The model under review builds one solid part; all positions refer to its coordinate system, in mm. Give positions to 0.01 mm unless a question says otherwise; leave off trailing zeros. Loops run counter-clockwise (first coordinate to the right, second up) from the corner with the lowest first, then second, coordinate; pieces in that order, holes last. Notation, with made-up numbers: (86.25, 21) -> (117.25, 21) arc R27 cw to (117.25, 60) -> close; hole circle Ø8 at (10, 67). An arc over 180 degrees is marked (long way). Write each question's results on one line, items separated by ' | '. Start each with the question number.
Q1. We need section B-B (x = 62). Write out the cut boundary in (y, z), plus the area to 3 significant figures.
Q2. Insertion check: pin 1 Ø1.8 at (y, z) = (-3.5, 5.5) entering from +X; pin 2 Ø3 at (x, y) = (133.5, -2) entering from -Z; pin 3 Ø2.5 at (y, z) = (-2.5, 222) entering from +X; pin 4 Ø6 at (x, z) = (76.5, 101.5) entering from +Y. Each pin has a flat end and moves straight along its axis. Give the tip position at first contact, or say it passes through.
Q3. Wall thickness on L1, parallel to X at y = -0.35, z = 2; L2, parallel to Z at x = 5, y = -3.1; L3, parallel to Z at x = 73, y = -4.35: over which ranges is each line inside the solid? List them lowest first. Write a range as [from, to].
Q4. We need section A-A (z = 106.5). Write out the cut boundary in (x, y), plus the area to 3 significant figures.
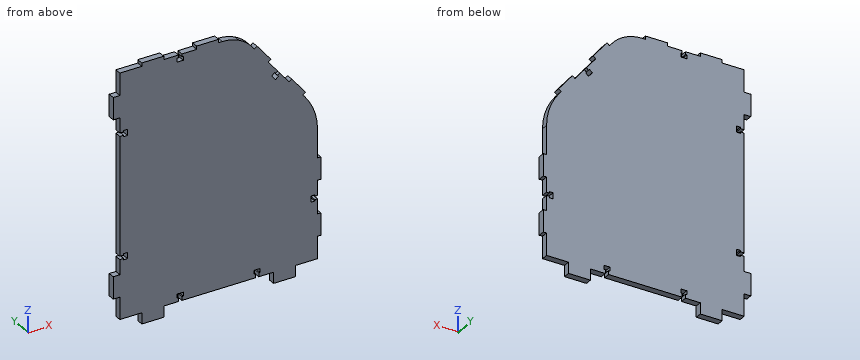
from build123d import *

# Parameters (mm, degrees)
F1_DEPTH = 6


# Not quite as in the source:
# - a feature names something its author has since deleted; it is built from what else it names


with BuildPart() as f1:
    # F0 (on Front) → F1 (new body)
    with BuildSketch(Plane.XZ):
        with BuildLine():
            Line((20, 220), (0, 220))
            Line((0, 220), (0, 200))
            Line((0, 200), (-6, 200))
            Line((-6, 200), (-6, 180))
            Line((-6, 180), (0, 180))
            Line((0, 180), (0, 166.5))
            Line((0, 166.5), (3.5, 166.5))
            Line((3.5, 166.5), (3.5, 167.75))
            Line((3.5, 167.75), (7, 167.75))
            Line((7, 167.75), (7, 162.25))
            Line((7, 162.25), (3.5, 162.25))
            Line((3.5, 162.25), (3.5, 163.5))
            Line((3.5, 163.5), (0, 163.5))
            Line((0, 163.5), (0, 110))
            Line((0, 110), (0, 56.5))
            Line((0, 56.5), (3.5, 56.5))
            Line((3.5, 56.5), (3.5, 57.75))
            Line((3.5, 57.75), (7, 57.75))
            Line((7, 57.75), (7, 52.25))
            Line((7, 52.25), (3.5, 52.25))
            Line((3.5, 52.25), (3.5, 53.5))
            Line((3.5, 53.5), (0, 53.5))
            Line((0, 53.5), (0, 40))
            Line((0, 40), (-6, 40))
            Line((-6, 40), (-6, 20))
            Line((-6, 20), (0, 20))
            Line((0, 20), (0, 0))
            Line((0, 0), (20, 0))
            Line((20, 0), (20, -10))
            Line((20, -10), (40, -10))
            Line((40, -10), (40, 0))
            Line((40, 0), (53.5, 0))
            Line((53.5, 0), (53.5, 3.5))
            Line((53.5, 3.5), (52.25, 3.5))
            Line((52.25, 3.5), (52.25, 7))
            Line((52.25, 7), (57.75, 7))
            Line((57.75, 7), (57.75, 3.5))
            Line((57.75, 3.5), (56.5, 3.5))
            Line((56.5, 3.5), (56.5, 0))
            Line((56.5, 0), (90, 0))
            Line((90, 0), (123.5, 0))
            Line((123.5, 0), (123.5, 3.5))
            Line((123.5, 3.5), (122.25, 3.5))
            Line((122.25, 3.5), (122.25, 7))
            Line((122.25, 7), (127.75, 7))
            Line((127.75, 7), (127.75, 3.5))
            Line((127.75, 3.5), (126.5, 3.5))
            Line((126.5, 3.5), (126.5, 0))
            Line((126.5, 0), (140, 0))
            Line((140, 0), (140, -10))
            Line((140, -10), (160, -10))
            Line((160, -10), (160, 0))
            Line((160, 0), (180, 0))
            Line((180, 0), (180, 20))
            Line((180, 20), (183, 20))
            Line((183, 20), (183, 40))
            Line((183, 40), (180, 40))
            Line((180, 40), (180, 53.5))
            Line((180, 53.5), (177.5, 53.5))
            Line((177.5, 53.5), (177.5, 52.25))
            Line((177.5, 52.25), (174, 52.25))
            Line((174, 52.25), (174, 57.75))
            Line((174, 57.75), (177.5, 57.75))
            Line((177.5, 57.75), (177.5, 56.5))
            Line((177.5, 56.5), (180, 56.5))
            Line((180, 56.5), (180, 70))
            Line((180, 70), (183, 70))
            Line((183, 70), (183, 90))
            Line((183, 90), (180, 90))
            Line((180, 90), (180, 110))
            Line((180, 110), (180, 116.0255279073))
            ThreePointArc((180, 116.0255279073), (177.1222639523, 132.7435493216), (168.8203103996, 147.5371686211))
            Line((168.8203103996, 147.5371686211), (166.7209532849, 150.1234412807))
            Line((166.7209532849, 150.1234412807), (169.0501719088, 152.0141397235))
            Line((169.0501719088, 152.0141397235), (156.4455156233, 167.5422638833))
            Line((156.4455156233, 167.5422638833), (154.1162969993, 165.6515654405))
            Line((154.1162969993, 165.6515654405), (145.6081540066, 176.1330492484))
            Line((145.6081540066, 176.1330492484), (143.6671384866, 174.5574672127))
            Line((143.6671384866, 174.5574672127), (144.4549295045, 173.5869594527))
            Line((144.4549295045, 173.5869594527), (141.7375077765, 171.3811446028))
            Line((141.7375077765, 171.3811446028), (138.271227298, 175.6513787467))
            Line((138.271227298, 175.6513787467), (140.988649026, 177.8571935967))
            Line((140.988649026, 177.8571935967), (141.7764400438, 176.8866858367))
            Line((141.7764400438, 176.8866858367), (143.7174555638, 178.4622678724))
            Line((143.7174555638, 178.4622678724), (135.2093125711, 188.9437516803))
            Line((135.2093125711, 188.9437516803), (137.538531195, 190.8344501231))
            Line((137.538531195, 190.8344501231), (124.9338749095, 206.362574283))
            Line((124.9338749095, 206.362574283), (122.6046562855, 204.4718758401))
            Line((122.6046562855, 204.4718758401), (120.5052991708, 207.0581484997))
            ThreePointArc((120.5052991708, 207.0581484997), (114.9751472562, 212.5051710496), (108.3804141438, 216.5993290869))
            ThreePointArc((108.3804141438, 216.5993290869), (101.0454672184, 219.1392480735), (93.331081891, 220))
            Line((93.331081891, 220), (90, 220))
            Line((90, 220), (90, 223))
            Line((90, 223), (70, 223))
            Line((70, 223), (70, 220))
            Line((70, 220), (56.5, 220))
            Line((56.5, 220), (56.5, 217.5))
            Line((56.5, 217.5), (57.75, 217.5))
            Line((57.75, 217.5), (57.75, 214))
            Line((57.75, 214), (52.25, 214))
            Line((52.25, 214), (52.25, 217.5))
            Line((52.25, 217.5), (53.5, 217.5))
            Line((53.5, 217.5), (53.5, 220))
            Line((53.5, 220), (40, 220))
            Line((40, 220), (40, 223))
            Line((40, 223), (20, 223))
            Line((20, 223), (20, 220))
        make_face()
    extrude(amount=F1_DEPTH)


solid = f1.part
Output:
1) outline: (-6, 0) -> (0, 0) -> (0, 220) -> (-6, 220) -> close | area: 1,320 mm2
2) pin 1: x = 180 | pin 2: z = 0 | pin 3: x = 90 | pin 4: y = 0
3) L1: [0, 53.5], [56.5, 123.5], [126.5, 180] | L2: [0, 52.25], [57.75, 162.25], [167.75, 220] | L3: [0, 223]
4) outline: (0, -6) -> (180, -6) -> (180, 0) -> (0, 0) -> close | area: 1,080 mm2
